```python
from build123d import *

# Parameters (mm, degrees)
SKETCH2_W          = 1.42
SKETCH2_H          = 2.84
SKETCH2_W_2        = 2.84
SKETCH2_H_2        = 1.42
CUT_EXTRUDE1_DEPTH = 3.85
DRAFT1_ANGLE       = 26.5
CHAMFER1_SIZE      = 0.5


with BuildPart() as part:
    # Sketch1 → Revolve1 (revolve)
    with BuildSketch(Plane.XY):
        with BuildLine():
            Line((-1.4, 5.65), (-2.05, 5.65))
            Line((-2.05, 5.65), (-4.7, 3))
            Line((-4.7, 3), (-21.4, 3))
            Line((-21.4, 3), (-21.4, 0))
            Line((-21.4, 0), (0, 0))
            ThreePointArc((0, 0), (-0.355213526, 2.910433816), (-1.4, 5.65))
        make_face()
    revolve(axis=Axis((0, 0, 0), (-1, 0, 0)))

    # Sketch2 → Cut-Extrude1 (cut)
    with BuildSketch(Plane(origin=(0, 0, 0), x_dir=(0, 0, -1), z_dir=(1, 0, 0))):
        with Locations((0, 2.13)):
            Rectangle(SKETCH2_W, SKETCH2_H)
        with Locations((-2.13, 0)):
            Rectangle(SKETCH2_W_2, SKETCH2_H_2)
        Rectangle(SKETCH2_W, SKETCH2_H_2)
        with Locations((2.13, 0)):
            Rectangle(SKETCH2_W_2, SKETCH2_H_2)
        with Locations((0, -2.13)):
            Rectangle(SKETCH2_W, SKETCH2_H)
    extrude(amount=-CUT_EXTRUDE1_DEPTH, mode=Mode.SUBTRACT)

    # Draft1
    draft1_faces = [part.faces().sort_by_distance(p)[0] for p in [
        (-2.194846815, -3.55, 0),
        (-2.194846815, 0, 3.55),
        (-2.194846815, 0, -3.55),
        (-2.194846815, 3.55, 0),
    ]]
    draft(draft1_faces, Plane(origin=(0, 0, 0), x_dir=(0, 0, 1), z_dir=(1, 0, 0)), DRAFT1_ANGLE)

    # Chamfer1
    chamfer1_edges = [part.edges().sort_by_distance(p)[0] for p in [
        (-21.4, -3, 0),
    ]]
    chamfer(chamfer1_edges, length=CHAMFER1_SIZE)


solid = part.part
```
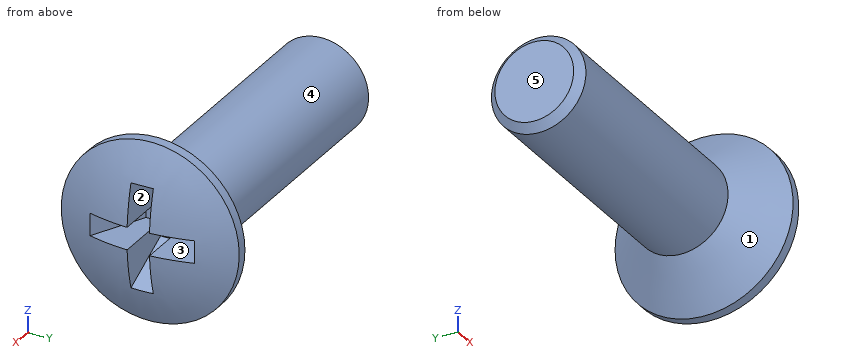
Geometry check sheet. Reference: the model listing, model coordinates, mm. Face numbers are marked on the shaded views. A direction names the side the tool comes from. Give positions to 0.01 mm unless a question says otherwise; leave off trailing zeros. Order: outer loops, then holes, each group sorted by start corner. A loop starts at its lowest first (then second) coordinate and runs counter-clockwise, first axis right, second up. Notation, with made-up numbers: (60, 30.5) - (113, 30.5) arc R28 cw to (113, 68.5) - close; hole circle Ø7 at (85, 7.25). An arc over 180 degrees is marked (long way). Answer in a Markdown table with one row per item. Add a question column.
Q1. Cross-section at D-D, the plane x = -7.5. Enter the section's corners in (y, z), then the cut area to 3 significant figures.
Q2. Mould release check, pull along Z, two halves, no side actions. Record for the marked faces 3, 4 and 5: pulls with the +Z half, pulls with the -Z half, needs draft (parallel to the pull), parting line crosses it, or undercut.
Q3. Tool access check on the marked faces 1 and 2. Record the directions out of +Z, -Z, +X, -X, +Y, -Y that give a thin tool (end or side, any length) a straight path to the whole face; none if there is none.
Q4. Cross-section at B-B, the plane x = -2.5. Enter the section's corners in (y, z).
Q5. Gauge pin test, flat ends, axial feed: pin 1 (6 mm diameter, centred on x = -5, z = -2.5, fed in from +Y); pin 2 (1.5 mm diameter, centred on y = -1.5, z = 3, fed in from -X); pin 3 (2 mm diameter, centred on x = -1.5, y = -1.5, fed in from -Z). Record the tip position at first contact, or that the pin passes through.
Q6. Cross-section at A-A, the plane y = 0. Enter the section's corners in (x, z).
Q7. Material ranges on probe 1 along Y at (x, z) = (-1.75, 2.5); probe 2 along X at (y, z) = (-2.25, 1); probe 3 along X at (y, z) = (-3, 4.25), recorded low to high. Write a range as from..to.
Check values:
| question | item | result |
|---|---|---|
| 1 | outline | circle Ø6 at (0, 0) |
| 1 | area | 28.3 mm^2 |
| 2 | face 3 | undercut |
| 2 | face 4 | parting line crosses it |
| 2 | face 5 | needs draft |
| 3 | face 1 | -X |
| 3 | face 2 | +X |
| 4 | outline | circle Ø10.4 at (0, 0); hole (-2.3, -0.71) - (-0.71, -0.71) - (-0.71, -2.3) - (0.71, -2.3) - (0.71, -0.71) - (2.3, -0.71) - (2.3, 0.71) - (0.71, 0.71) - (0.71, 2.3) - (-0.71, 2.3) - (-0.71, 0.71) - (-2.3, 0.71) - close |
| 5 | pin 1 | stops at y = 5.33 |
| 5 | pin 2 | stops at x = -21.3 |
| 5 | pin 3 | stops at z = -5.63 |
| 6 | outline | (-21.4, -2.5) - (-20.9, -3) - (-4.7, -3) - (-2.05, -5.65) - (-1.4, -5.65) arc R12.1 ccw to (-0.46, -3.32) - (-3.85, -1.63) - (-3.85, 1.63) - (-0.46, 3.32) arc R12.1 ccw to (-1.4, 5.65) - (-2.05, 5.65) - (-4.7, 3) - (-20.9, 3) - (-21.4, 2.5) - close |
| 7 | probe 1 | y = -5.07..-0.71, 0.71..5.07 |
| 7 | probe 2 | x = -21.4..-0.25 |
| 7 | probe 3 | x = -2.5..-1.18 |
